Here's how the part is built. I have some questions about the finished solid (model axes, mm). A direction names the side the tool comes from. Round coordinates to 2 decimals unless told otherwise and drop trailing zeros. Order: outer loops, then holes, each group sorted by start corner. A loop starts at its lowest first (then second) coordinate and runs counter-clockwise, first axis right, second up. Notation, with made-up numbers: M 7,-39.75 L 20,-39.75 A16 ccw 20,-31.75 Z; hole C 31.5,33.5 d8. An arc over 180 degrees is marked long. Write item = value, one per line. Start each with the question number.
Item 1: Please list where these lines run through material, in increasing order: L1, parallel to X at y = 2.25, z = 8.5 (3 decimals); L2, parallel to X at y = 0.95, z = -16.51 (1 decimal); L3, parallel to Y at x = -21.5, z = -14.
Item 2: I want a section at A-A, the plane y = 8.5. List the corners of the cut face in (x, z) for me.
Item 3: I'm going to push flat-ended pins straight in: P1, Ø3, axis at y = 4.5, z = -0.5, coming from the +X side; P2, Ø11, axis at x = 22.5, z = 8, coming from the +Y side; P3, Ø4, axis at x = 26.035, z = -16.51, coming from the -Y side; P4, Ø1.9, axis at x = -26.543, z = -17.018, coming from the +Y side. Where does each tip first touch, or does it pass through?
Item 4: We'd pull the mould along Z, two halves only. Please class faces 1 (the face through (-24, 7, 8.128)), 2 (the face through (19, 3.734, 11)), 3 (the face through (-10, 1, -20.32)): pulls with the +Z half, pulls with the -Z half, needs draft (parallel to the pull), parting line crosses it, or undercut.
Item 5: For faces 4 (the face through (-24, 7, -5.334)), 5 (the face through (24, 1, -20.32)), 6 (the face through (-28.067, 7, 13)), 7 (the face through (19, 3, 2.54)), 8 (the face through (-20.701, 7, 13)), which set-ups out of +Z, -Z, +X, -X, +Y, -Y let a thin tool reach every point of the face, with its end or its side?
Item 6: I want a section at B-B, the plane z = 0. List the corners of the cut face in (x, y) for me (3 decimals), plus the area to 3 significant figures.
Item 7: I want a section at C-C, the plane x = 17. List the corners of the cut face in (y, z) for me.
Item 8: I want a section at D-D, the plane y = 0.75. List the corners of the cut face in (x, z) for me (1 decimal).
```python
from build123d import *

# Parameters (mm, degrees)
SKETCH1_W           = 59.69
SKETCH1_H           = 40.64
SKETCH1_R           = 1.5875
BOSS_EXTRUDE1_DEPTH = 1.6256
SKETCH2_W           = 13.97
SKETCH2_H           = 17.78
BOSS_EXTRUDE2_DEPTH = 2.1082
BOSS_EXTRUDE3_START = 1.016
SKETCH3_W           = 6.604
SKETCH3_H           = 17.526
BOSS_EXTRUDE3_DEPTH = 6.35
SKETCH4_W           = 7.366
SKETCH4_H           = 9.652
BOSS_EXTRUDE4_DEPTH = 10.16


with BuildPart() as part:
    # Sketch1 → Boss-Extrude1 (new body)
    with BuildSketch(Plane(origin=(0, 0, 0), x_dir=(1, 0, 0), z_dir=(0, 1, 0))):
        Rectangle(SKETCH1_W, SKETCH1_H)
        with Locations(Location((26.035, 16.51, 0), (0, 0, 270))):
            Circle(SKETCH1_R, mode=Mode.SUBTRACT)
        with Locations(Location((-26.543, 17.018, 0), (0, 0, 270))):
            Circle(SKETCH1_R, mode=Mode.SUBTRACT)
    extrude(amount=BOSS_EXTRUDE1_DEPTH)

    # Sketch2 → Boss-Extrude2 (add)
    with BuildSketch(Plane(origin=(0, 1.6256, 0), x_dir=(1, 0, 0), z_dir=(0, 1, 0))):
        with Locations((19.05, -11.43)):
            Rectangle(SKETCH2_W, SKETCH2_H)
    extrude(amount=BOSS_EXTRUDE2_DEPTH)

    # Sketch3 → Boss-Extrude3 (add)
    with BuildSketch(Plane(origin=(0, 1.6256, 0), x_dir=(1, 0, 0), z_dir=(0, 1, 0)).offset(BOSS_EXTRUDE3_START)):
        with Locations((14.605, 25.019)):
            Rectangle(SKETCH3_W, SKETCH3_H)
    extrude(amount=-BOSS_EXTRUDE3_DEPTH)

    # Sketch4 → Boss-Extrude4 (add)
    with BuildSketch(Plane(origin=(0, 1.6256, 0), x_dir=(1, 0, 0), z_dir=(0, 1, 0))):
        with Locations((-24.384, -12.954)):
            Rectangle(SKETCH4_W, SKETCH4_H)
        with Locations((-24.384, 0.508)):
            Rectangle(SKETCH4_W, SKETCH4_H)
    extrude(amount=BOSS_EXTRUDE4_DEPTH)


solid = part.part
```
Filled in:
q1.L1 = -28.067 to -20.701, 12.065 to 26.035
q1.L2 = -29.8 to -28, -25 to 24.4, 27.6 to 29.8
q1.L3 = 0 to 1.63
q2.outline = M -28.07,-5.33 L -20.7,-5.33 L -20.7,4.32 L -28.07,4.32 Z; M -28.07,8.13 L -20.7,8.13 L -20.7,17.78 L -28.07,17.78 Z
q3.P1 = -20.7
q3.P2 = 3.73
q3.P3 = 0
q3.P4 = through
q4.face_1 = undercut
q4.face_2 = needs draft
q4.face_3 = pulls with the -Z half
q5.face_4 = -Z, +X, -X, +Y
q5.face_5 = -Z, +X, +Y, -Y
q5.face_6 = +Z, -Z, -X, +Y
q5.face_7 = +X, +Y
q5.face_8 = +Z, -Z, +Y
q6.outline = M -29.845,0 L 29.845,0 L 29.845,1.626 L -20.701,1.626 L -20.701,11.786 L -28.067,11.786 L -28.067,1.626 L -29.845,1.626 Z
q6.area = 172 mm^2
q7.outline = M -3.71,-33.78 L 2.64,-33.78 L 2.64,-16.26 L 1.63,-16.26 L 1.63,2.54 L 3.73,2.54 L 3.73,20.32 L 0,20.32 L 0,-16.26 L -3.71,-16.26 Z
q8.outline = M -29.8,-20.3 L 11.3,-20.3 L 11.3,-33.8 L 17.9,-33.8 L 17.9,-20.3 L 29.8,-20.3 L 29.8,20.3 L -29.8,20.3 Z; hole C -26.5,-17 d3.2; hole C 26,-16.5 d3.2
